```python
from build123d import *

# Parameters (mm, degrees)
F0_R            = 46
F0_R_2          = 20.5
F1_DEPTH        = 3
F2_W            = 2
F2_H            = 3
F3_DEPTH        = 3
F3_COPIES_COUNT = 30


# Not quite as in the source:
# - a pattern or mirror of a feature is missing from the dataset's text; its kind, count and spacing are read off the source's solid


with BuildPart() as f1:
    # F0 (on Front) → F1 (new body)
    with BuildSketch(Plane.XZ):
        Circle(F0_R)
        Circle(F0_R_2, mode=Mode.SUBTRACT)
    extrude(amount=F1_DEPTH)

    # F2 (on Front) → F3 (cut)
    with BuildSketch(Plane.XZ):
        with Locations((-45, 0)):
            Rectangle(F2_W, F2_H)
    f3 = extrude(amount=F3_DEPTH, mode=Mode.SUBTRACT)

    # F3_copies: F3 ×30 about axis
    f3_copies_axis = Axis((0, 0, 0), (0, 1, 0))
    for i in range(1, F3_COPIES_COUNT):
        add(f3.rotate(f3_copies_axis, i * 360 / F3_COPIES_COUNT), mode=Mode.SUBTRACT)


solid = f1.part
```
The model under review builds one solid part; all positions refer to its coordinate system, in mm. A direction names the side the tool comes from. Round coordinates to 2 decimals unless told otherwise and drop trailing zeros. Loops run counter-clockwise (first coordinate to the right, second up) from the corner with the lowest first, then second, coordinate; pieces in that order, holes last. Notation, with made-up numbers: (5, 59.5) - (14, 59.5) arc R19 cw to (14, 67.5) - close; hole circle Ø7 at (-2, 22.25). An arc over 180 degrees is marked (long way). Use a Markdown table: item, result. Add a question column.
Q1. Add section A-A (z = 0). State the section outline as (x, y) points, plus the area to 3 significant figures.
Q2. Insertion check: pin 1 Ø4 at (x, z) = (33.5, -35.5) entering from +Y; pin 2 Ø1 at (x, y) = (-35.5, -0.5) entering from +Z. Each pin has a flat end and moves straight along its axis. Give the tip position at first contact, or say it passes through.
Q3. The part is to be moulded in two halves that separate along X. For faces 1 (the face through (45.743, -1.479, -4.854)), 2 (the face through (-35.609, -1.479, 25.846)), 3 (the face through (-45, -1, -1.5)), say which applies: pulls with the +X half, pulls with the -X half, needs draft (parallel to the pull), parting line crosses it, or undercut.
Q4. Add section C-C (x = 33). State the section outline as (y, z) points, plus the area to 3 significant figures.
Q5. For probe 1 along Z at (x, y) = (0, -0.8); probe 2 along Z at (x, y) = (35, -2.1); probe 3 along X at (y, z) = (-1, 1), list the stretches that pass through material, from the lowest coordinate up.
Q6. Machinability: for faces 4 (the face through (-44, -1, 0)), 5 (the face through (-18.67, -1.48, 42.04)), 6 (the face through (-40.187, -1.479, -17.916)), 7 (the face through (45, -1, 1.5)), which of the approach directions +Z, -Z, +X, -X, +Y, -Y give a long, thin tool a straight path to every point of the face, cutting with its end or side? Answer none if there is none.
Q7. Add section B-B (x = -9). State the section outline as (y, z) points.
Worked answers:
| question | item | result |
|---|---|---|
| 1 | outline | (-44, -3) - (-20.5, -3) - (-20.5, 0) - (-44, 0) - close; (20.5, -3) - (44, -3) - (44, 0) - (20.5, 0) - close |
| 1 | area | 141 mm² |
| 2 | pin 1 | through |
| 2 | pin 2 | z = 29.85 |
| 3 | face 1 | pulls with the +X half |
| 3 | face 2 | undercut |
| 3 | face 3 | needs draft |
| 4 | outline | (-3, -32.05) - (0, -32.05) - (0, 32.05) - (-3, 32.05) - close |
| 4 | area | 192 mm² |
| 5 | probe 1 | -46 to -20.5, 20.5 to 46 |
| 5 | probe 2 | -29.85 to -27.28, -26.68 to 26.68, 27.28 to 29.85 |
| 5 | probe 3 | -44 to -20.48, 20.48 to 44 |
| 6 | face 4 | -X, +Y, -Y |
| 6 | face 5 | +Z, -X, +Y, -Y |
| 6 | face 6 | +Y, -Y |
| 6 | face 7 | +X, +Y, -Y |
| 7 | outline | (-3, -45.11) - (0, -45.11) - (0, -18.42) - (-3, -18.42) - close; (-3, 18.42) - (0, 18.42) - (0, 45.11) - (-3, 45.11) - close |
